Geometry check sheet. Reference: the model listing, model coordinates, mm. Face numbers are marked on the shaded views. A direction names the side the tool comes from. Give positions to 0.01 mm unless a question says otherwise; leave off trailing zeros. Loops run counter-clockwise (first coordinate to the right, second up) from the corner with the lowest first, then second, coordinate; pieces in that order, holes last. Notation, with made-up numbers: (18, -36.75) -> (49, -36.75) arc R34 cw to (49, -3.75) -> close; hole circle Ø4 at (51.5, 52). An arc over 180 degrees is marked (long way). Write each question's results on one line, items separated by ' | '. Start each with the question number.
1) Sectioned sample at B-B on z = -1.75. Record the cut outline in (x, y).
2) Depth check by flat-ended pin: pin 1 (0.6 mm diameter, centred on y = -5.5, z = 3.5, fed in from -X); pin 2 (3.5 mm diameter, centred on y = -6, z = 4.5, fed in from +X); pin 3 (4 mm diameter, centred on x = 3, y = -3.5, fed in from +Z). Enter the tip coordinate at first touch or a pass-through.
3) Sectioned sample at A-A on y = -9. Record the cut outline in (x, z), then the cut area to 3 significant figures.
4) Scan lines: line 1 (X direction, y = -0.5, z = -6.75); line 2 (Z direction, x = 1.5, y = -8); line 3 (X direction, y = -3.75, z = 5.75). Record each from-to range of solid material in increasing order. Write a range as from..to.
5) Sectioned sample at C-C on x = 2. Record the cut outline in (y, z), then the cut area to 3 significant figures.
6) Set-up check for the marked faces 1, 2, 3 and 4: record each of +Z, -Z, +X, -X, +Y, -Y from which the full face is reachable in a straight line by a thin tool's end or side.
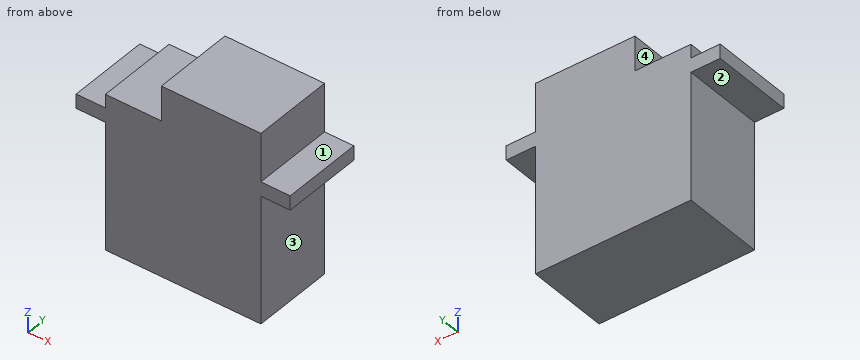
```python
from build123d import *

# Parameters (mm, degrees)
F0_W     = 22.8
F0_H     = 18.7
F0_W_2   = 4.3
F0_H_2   = 2.1
F0_W_3   = 14.6
F0_H_3   = 5.1
F1_DEPTH = 12


with BuildPart() as f1:
    # F0 (on Front) → F1 (new body)
    with BuildSketch(Plane.XZ):
        with Locations((11.4, -9.35)):
            Rectangle(F0_W, F0_H)
        with Locations((-2.15, 1.05)):
            Rectangle(F0_W_2, F0_H_2)
        Polygon((8.2, 4.1), (0, 4.1), (0, 2.1), (22.8, 2.1), (22.8, 4.1), align=None)
        with Locations((11.4, 1.05)):
            Rectangle(F0_W, F0_H_2)
        with Locations((15.5, 6.65)):
            Rectangle(F0_W_3, F0_H_3)
        with Locations((24.95, 1.05)):
            Rectangle(F0_W_2, F0_H_2)
    extrude(amount=F1_DEPTH)


solid = f1.part
```
Result:
1) outline: (0, -12) -> (22.8, -12) -> (22.8, 0) -> (0, 0) -> close
2) pin 1: x = 0 | pin 2: x = 22.8 | pin 3: z = 4.1
3) outline: (-4.3, 0) -> (0, 0) -> (0, -18.7) -> (22.8, -18.7) -> (22.8, 0) -> (27.1, 0) -> (27.1, 2.1) -> (22.8, 2.1) -> (22.8, 9.2) -> (8.2, 9.2) -> (8.2, 4.1) -> (0, 4.1) -> (0, 2.1) -> (-4.3, 2.1) -> close | area: 612 mm^2
4) line 1: 0..22.8 | line 2: -18.7..4.1 | line 3: 8.2..22.8
5) outline: (-12, -18.7) -> (0, -18.7) -> (0, 4.1) -> (-12, 4.1) -> close | area: 274 mm^2
6) face 1: +Z, +X, +Y, -Y | face 2: -Z, -X, +Y, -Y | face 3: -Z, +X, +Y, -Y | face 4: +Z, -X, +Y, -Y
